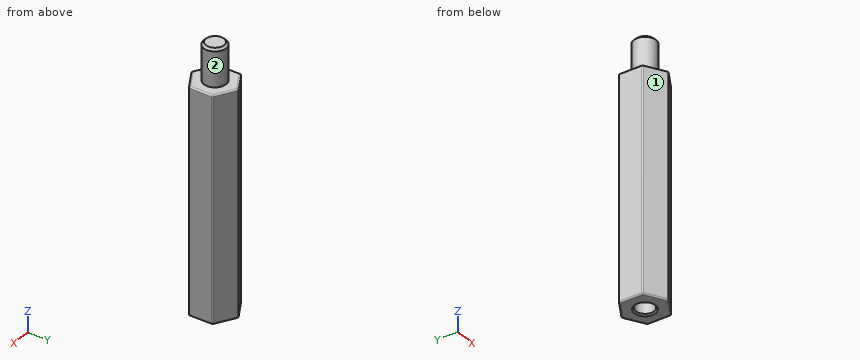
Autodesk Inventor part; units mm, degrees
ref_plane "YZ Plane" through (0, 0, 0) normal (1, 0, 0) x (0, 1, 0)
ref_plane "XZ Plane" through (0, 0, 0) normal (0, 1, 0) x (-1, 0, 0)
ref_plane "XY Plane" through (0, 0, 0) normal (0, 0, 1) x (1, 0, 0)
sketch "スケッチ1" plane through (0, 0, 0) normal (0, 0, 1) x (1, 0, 0)
  line L0 (0, 3.1754) -> (2.75, 1.5877)
  line L1 (2.75, 1.5877) -> (2.75, -1.5877)
  line L2 (2.75, -1.5877) -> (0, -3.1754)
  line L3 (0, -3.1754) -> (-2.75, -1.5877)
  line L4 (-2.75, -1.5877) -> (-2.75, 1.5877)
  line L5 (-2.75, 1.5877) -> (0, 3.1754)
  point P0 (0, 0)
  point P1 (0, 0)
  dimension "d0" = 5.5
extrude "押し出し1" add sketch "スケッチ1" along normal blind 30
sketch "スケッチ2" plane through (0, 0, 30) normal (0, 0, 1) x (1, 0, 0)
  circle A0 centre (0, 0) radius 1.5
  dimension "d3" = 3
extrude "押し出し2" add sketch "スケッチ2" along normal blind 5
thread "ねじ1"
chamfer "面取り1" distance 0.3 angle 45 1 edges at (-1.5, 0, 35)
fillet "フィレット1" radius 0.2 18 edges at (-1.375, 2.3816, 30) (1.375, 2.3816, 30) (2.75, 0, 30) (1.375, -2.3816, 30) (-1.375, -2.3816, 30) (-2.75, 0, 30) (-2.75, -1.5877, 15) (0, -3.1754, 15) (2.75, -1.5877, 15) (2.75, 1.5877, 15) (0, 3.1754, 15) (-2.75, 1.5877, 15) (-1.375, 2.3816, 0) (1.375, 2.3816, 0) (2.75, 0, 0) (1.375, -2.3816, 0) (-1.375, -2.3816, 0) (-2.75, 0, 0)
sketch "スケッチ3" plane through (0, 0, 0) normal (0, 0, -1) x (-1, 0, 0)
  point P0 (0, 0)
hole "穴1" at (0, 0, 0) direction (0, 0, 1) diameter 2.459 depth 5 tip angle 118
chamfer "面取り2" distance 0.2 angle 45 1 edges at (0, -1.2295, 0)
properties part number "hexagonal_spacer_M3_30mm" material "鋼、炭素鋼"
Source: CAD feature listing. Evaluate the final solid. Frame: model axes, mm. Face numbers are marked on the shaded views. A direction names the side the tool comes from. Give positions to 0.01 mm unless a question says otherwise; leave off trailing zeros. Order: outer loops, then holes, each group sorted by start corner. A loop starts at its lowest first (then second) coordinate and runs counter-clockwise, first axis right, second up.
(1) Material intervals for line 1 along Y through (x, z) = (0, 1.25); line 2 along X through (y, z) = (0, 1.85); line 3 along Z through (x, y) = (-1.8, -1.5), sorted ascending.
(2) Section query A-A (z = 19.5). Return the cut outline in (x, y), plus the area to 3 significant figures.
(3) Access query for the marked faces 1 and 2. Directions: +Z, -Z, +X, -X, +Y, -Y. A direction counts if a zero-diameter tool reaches every point of the face in a straight line with its end or side. Return the directions, or none.
Outcome:
1. line 1: y = -3.14 to -1.23, 1.23 to 3.14
1. line 2: x = -2.75 to -1.23, 1.23 to 2.75
1. line 3: z = 0 to 30
2. outline: (-2.75, -1.47) arc R0.2 ccw to (-2.65, -1.65) - (-0.1, -3.12) arc R0.2 ccw to (0.1, -3.12) - (2.65, -1.65) arc R0.2 ccw to (2.75, -1.47) - (2.75, 1.47) arc R0.2 ccw to (2.65, 1.65) - (0.1, 3.12) arc R0.2 ccw to (-0.1, 3.12) - (-2.65, 1.65) arc R0.2 ccw to (-2.75, 1.47) - close
2. area: 26.2 mm2
3. face 1: +Z, -Z, -X, -Y
3. face 2: +Z
